Source: CAD feature listing. Evaluate the final solid. Frame: model axes, mm. A direction names the side the tool comes from. Round coordinates to 2 decimals unless told otherwise and drop trailing zeros. Write each loop counter-clockwise with the first axis right and the second up, starting at its lowest first coordinate (ties: lowest second). Pieces come first, ordered by that corner, then holes. Notation, with made-up numbers: M 36,54.25 L 49,54.25 A14 ccw 49,75.25 Z; hole C -28,46 d3. An arc over 180 degrees is marked long. Put each result on its own line as item: value. Start each with the question number.
```python
from build123d import *

# Parameters (mm, degrees)
F0_W     = 5
F0_H     = 47.625
F0_W_2   = 146.05
F0_R     = 3.24
F1_DEPTH = 50
F2_W     = 119.824
F2_H     = 42.025
F3_DEPTH = 45
F4_D     = 5.6
F4_DEPTH = 20
F4_TIP   = 1.6824097333
F5_W     = 40
F5_H     = 5
F6_DEPTH = 47.626
F7_D     = 4


# Not quite as in the source:
# - ends of sketch curves that miss each other by under 0.0002 mm in the source are joined


with BuildPart() as f1:
    # F0 (on Top) → F1 (new body)
    with BuildSketch(Plane.XY):
        with Locations((-75.525, 0)):
            Rectangle(F0_W, F0_H)
        Rectangle(F0_W_2, F0_H)
        with Locations((-68.262, -9.5245)):
            Circle(F0_R, mode=Mode.SUBTRACT)
        with Locations((68.262, -9.5245)):
            Circle(F0_R, mode=Mode.SUBTRACT)
        with Locations((-68.262, 9.5245)):
            Circle(F0_R, mode=Mode.SUBTRACT)
        with BuildLine():
            Line((72.225, -15.859485), (72.225, -23.0125))
            Line((72.225, -23.0125), (-72.225, -23.0125))
            Line((-72.225, -23.0125), (-72.225, -15.874133))
            Line((-72.225, -15.874133), (-68.193705, -15.874133))
            ThreePointArc((-68.193705, -15.874133), (-61.912367271, -9.4562050029), (-68.3302949971, -3.174867271))
            Line((-68.3302949971, -3.174867271), (-72.225, -3.174867))
            Line((-72.225, -3.174867), (-72.225, 3.1745))
            Line((-72.225, 3.1745), (-68.262, 3.1745))
            ThreePointArc((-68.262, 3.1745), (-61.912, 9.5245), (-68.262, 15.8745))
            Line((-68.262, 15.8745), (-72.225, 15.8745))
            Line((-72.225, 15.8745), (-72.225, 23.0125))
            Line((-72.225, 23.0125), (72.225, 23.0125))
            Line((72.225, 23.0125), (72.225, 15.8745))
            Line((72.225, 15.8745), (68.262, 15.8745))
            ThreePointArc((68.262, 15.8745), (61.912, 9.5245), (68.262, 3.1745))
            Line((68.262, 3.1745), (72.225, 3.1745))
            Line((72.225, 3.1745), (72.225, -3.189515))
            Line((72.225, -3.189515), (67.825573, -3.189515))
            ThreePointArc((67.825573, -3.189515), (61.9270152731, -9.9609269812), (68.6984269812, -15.8594847269))
            Line((68.6984269812, -15.8594847269), (72.225, -15.859485))
        make_face(mode=Mode.SUBTRACT)
        with Locations((68.262, 9.5245)):
            Circle(F0_R, mode=Mode.SUBTRACT)
        with Locations((75.525, 0)):
            Rectangle(F0_W, F0_H)
        with Locations((-68.262, 9.5245)):
            Circle(F0_R)
        with Locations((-68.262, -9.5245)):
            Circle(F0_R)
        with BuildLine():
            Line((-72.225, -23.0125), (72.225, -23.0125))
            Line((72.225, -23.0125), (72.225, -15.859485))
            Line((72.225, -15.859485), (68.698427, -15.859485))
            ThreePointArc((68.698427, -15.859485), (61.9270152731, -9.9609269812), (67.8255730188, -3.1895152731))
            Line((67.8255730188, -3.1895152731), (72.225, -3.189515))
            Line((72.225, -3.189515), (72.225, 3.1745))
            Line((72.225, 3.1745), (68.262, 3.1745))
            ThreePointArc((68.262, 3.1745), (61.912, 9.5245), (68.262, 15.8745))
            Line((68.262, 15.8745), (72.225, 15.8745))
            Line((72.225, 15.8745), (72.225, 23.0125))
            Line((72.225, 23.0125), (-72.225, 23.0125))
            Line((-72.225, 23.0125), (-72.225, 15.8745))
            Line((-72.225, 15.8745), (-68.262, 15.8745))
            ThreePointArc((-68.262, 15.8745), (-61.912, 9.5245), (-68.262, 3.1745))
            Line((-68.262, 3.1745), (-72.225, 3.1745))
            Line((-72.225, 3.1745), (-72.225, -3.174867))
            Line((-72.225, -3.174867), (-68.330295, -3.174867))
            ThreePointArc((-68.330295, -3.174867), (-61.912367271, -9.4562050029), (-68.1937050029, -15.874132729))
            Line((-68.1937050029, -15.874132729), (-72.225, -15.874133))
            Line((-72.225, -15.874133), (-72.225, -23.0125))
        make_face()
        with Locations((68.262, 9.5245)):
            Circle(F0_R)
        with Locations((68.262, -9.5245)):
            Circle(F0_R)
    extrude(amount=-F1_DEPTH)

    # F2 (on face) → F3 (cut)
    with BuildSketch(Plane.XY):
        Rectangle(F2_W, F2_H)
    extrude(amount=-F3_DEPTH, mode=Mode.SUBTRACT)

    # F4
    with Locations(Plane.XY):
        with Locations((-68.262, 9.5245), (-68.262, -9.5245), (68.262, 9.5245), (68.262, -9.5245)):
            Hole(F4_D / 2, depth=F4_DEPTH)
            with Locations((0, 0, -(F4_DEPTH + F4_TIP / 2))):  # 118° drill point
                Cone(0, F4_D / 2, F4_TIP, mode=Mode.SUBTRACT)

    # F5 (on face) → F6 (cut, through all)
    with BuildSketch(Plane.XZ.offset(23.8125)):
        with Locations((0, -42.5)):
            Rectangle(F5_W, F5_H)
    extrude(amount=-F6_DEPTH, mode=Mode.SUBTRACT)

    # F7 (through all)
    with Locations(Plane.XZ.offset(23.8125)):
        with Locations((-49.912, -25), (49.912, -25)):
            Hole(F7_D / 2)


solid = f1.part
```
(1) Section query A-A (z = -25). Return loops of the section in (x, y) (1 decimal).
(2) Section query B-B (x = -28.5). Return loops of the section in (y, z).
(3) Section query D-D (x = 3.5). Return loops of the section in (y, z), and give its area (3 significant figures).
(4) Access query for faces 4 (the flat face through (0, -22, -40)), 5 (the flat face through (1, 23.812, -25)), 6 (the flat face through (-59.912, 0, -22)). Directions: +Z, -Z, +X, -X, +Y, -Y. A direction counts if a zero-diameter tool reaches every point of the face in a straight line with its end or side. Return the directions, or none.
(5) Pull-direction query (Z, two-part tool) for faces 1 (the conical face through (-68.75, 9.55, -21.39)), 2 (the flat face through (78.025, 0, -25)), 3 (the flat face through (-20, 22, -43)); classes: +Z half, -Z half, draft (parallel to the pull), parting line (faces both ways), or undercut.
(6) Contact query for a flat-ended pin moving along its axis: P1, Ø3.5, axis at x = 49.912, z = -25, coming from the +Y side. Output: stop coordinate, or through.
(7) Ray query, line 1 along Y through (x, z) = (-51, -22); line 2 along X through (y, z) = (10.5, -34) (3 decimals); line 3 along X through (y, z) = (-11, -2.5) (3 decimals). Return the intervals inside material, ascending.
(8) Section query C-C (y = -4.5). Return loops of the section in (x, z) (3 decimals), and give its area (3 significant figures).
Entries:
1. outline: M -78,-23.8 L -51.9,-23.8 L -51.9,-21 L -59.9,-21 L -59.9,21 L -51.9,21 L -51.9,23.8 L -78,23.8 Z; M -47.9,-23.8 L 47.9,-23.8 L 47.9,-21 L -47.9,-21 Z; M -47.9,21 L 47.9,21 L 47.9,23.8 L -47.9,23.8 Z; M 51.9,-23.8 L 78,-23.8 L 78,23.8 L 51.9,23.8 L 51.9,21 L 59.9,21 L 59.9,-21 L 51.9,-21 Z
2. outline: M -23.81,-50 L 23.81,-50 L 23.81,0 L 21.01,0 L 21.01,-45 L -21.01,-45 L -21.01,0 L -23.81,0 Z
3. outline: M -23.81,-50 L 23.81,-50 L 23.81,-45 L -23.81,-45 Z; M -23.81,-40 L -21.01,-40 L -21.01,0 L -23.81,0 Z; M 21.01,-40 L 23.81,-40 L 23.81,0 L 21.01,0 Z
3. area: 462 mm2
4. face 4: +Y, -Y
4. face 5: +Z, -Z, +X, -X, +Y
4. face 6: +Z
5. face 1: +Z half
5. face 2: draft
5. face 3: undercut
6. P1: through
7. line 1: -23.81 to -21.01, 21.01 to 23.81
7. line 2: -78.025 to -59.912, 59.912 to 78.025
7. line 3: -78.025 to -70.642, -65.882 to -59.912, 59.912 to 65.882, 70.642 to 78.025
8. outline: M -78.025,-50 L 78.025,-50 L 78.025,0 L 59.912,0 L 59.912,-45 L -59.912,-45 L -59.912,0 L -78.025,0 Z
8. area: 2,410 mm2
